Read the model definition and answer for the solid it produces. Units are mm, in the model's axes. A direction names the side the tool comes from. Give positions to 0.01 mm unless a question says otherwise; leave off trailing zeros. Write each loop counter-clockwise with the first axis right and the second up, starting at its lowest first coordinate (ties: lowest second). Pieces come first, ordered by that corner, then holes. Notation, with made-up numbers: (79.5, -9.75) - (136.5, -9.75) arc R33 cw to (136.5, 27.25) - close; hole circle Ø3 at (-18, 61.5). An arc over 180 degrees is marked (long way). Answer as a JSON object with one key per item and string values. Group by question number.
```python
from build123d import *

# Parameters (mm, degrees)
BOSS_EXTRUDE1_DEPTH     = 2
CUT_EXTRUDE1_DEPTH      = 6.766281297
CUT_EXTRUDE1_DEPTH_BACK = 6.766281297
SKETCH2_R               = 1.55
BOSS_EXTRUDE2_START     = 4.6
BOSS_EXTRUDE2_DEPTH     = 4.6
BOSS_EXTRUDE3_DEPTH     = 2
FILLET1_R               = 0.5


with BuildPart() as part:
    # Sketch1 → Boss-Extrude1 (new body)
    with BuildSketch(Plane(origin=(0, 0, 0), x_dir=(1, 0, 0), z_dir=(0, 1, 0))):
        with BuildLine():
            Line((2.5, 3), (-2.5, 3))
            ThreePointArc((-2.5, 3), (-3.914213562, 2.414213562), (-4.5, 1))
            Line((-4.5, 1), (-4.5, -1))
            ThreePointArc((-4.5, -1), (-3.914213562, -2.414213562), (-2.5, -3))
            Line((-2.5, -3), (2.5, -3))
            ThreePointArc((2.5, -3), (3.914213562, -2.414213562), (4.5, -1))
            Line((4.5, -1), (4.5, 1))
            ThreePointArc((4.5, 1), (3.914213562, 2.414213562), (2.5, 3))
        make_face()
    extrude(amount=BOSS_EXTRUDE1_DEPTH)

    # Sketch2 → Cut-Extrude1 (cut, two sides: drawn at the far end of the back side and taken through both)
    with BuildSketch(Plane(origin=(0, 2, 0), x_dir=(1, 0, 0), z_dir=(0, 1, 0)).offset(-CUT_EXTRUDE1_DEPTH_BACK)):
        with Locations(Location((-1.6, 0, 0), (0, 0, 270))):
            Circle(SKETCH2_R)
    extrude(amount=CUT_EXTRUDE1_DEPTH + CUT_EXTRUDE1_DEPTH_BACK, mode=Mode.SUBTRACT)

    # Sketch3 → Boss-Extrude2 (add)
    with BuildSketch(Plane.XZ.offset(BOSS_EXTRUDE2_START)):
        with BuildLine():
            Line((4.5, 1), (4.5, -1))
            ThreePointArc((4.5, -1), (3.914213562, -2.414213562), (2.5, -3))
            Line((2.5, -3), (2.5, 3))
            ThreePointArc((2.5, 3), (3.914213562, 2.414213562), (4.5, 1))
        make_face()
    extrude(amount=-BOSS_EXTRUDE2_DEPTH)

    # Sketch4 → Boss-Extrude3 (add)
    with BuildSketch(Plane.XZ.offset(4.6)):
        with BuildLine():
            Line((4.5, 1), (4.5, -1))
            ThreePointArc((4.5, -1), (3.914213562, -2.414213562), (2.5, -3))
            Line((2.5, -3), (5.5, -3))
            ThreePointArc((5.5, -3), (6.560660172, -2.560660172), (7, -1.5))
            Line((7, -1.5), (7, 1.5))
            ThreePointArc((7, 1.5), (6.560660172, 2.560660172), (5.5, 3))
            Line((5.5, 3), (2.5, 3))
            ThreePointArc((2.5, 3), (3.914213562, 2.414213562), (4.5, 1))
        make_face()
    extrude(amount=-BOSS_EXTRUDE3_DEPTH)

    # Fillet1
    # the kernel refuses this fillet: 0.5 mm, written as the material it takes off along each edge
    with BuildSketch(Plane(origin=(-2.5, 2, 1), x_dir=(-1, 0, 0), z_dir=(0, 0, -1))) as fillet1_piece_1:
        with BuildLine():
            CenterArc((2 - FILLET1_R, -FILLET1_R), FILLET1_R, 0, 90)
            Line((2, -FILLET1_R), (2, 0))
            Line((2, 0), (2 - FILLET1_R, 0))
        make_face()
    revolve(axis=Axis((-2.5, 2, 1), (0, 1, 0)), revolution_arc=90, mode=Mode.SUBTRACT)
    with BuildSketch(Plane(origin=(-2.5, 2, 3), x_dir=(0, 0, -1), z_dir=(1, 0, 0)), Plane(origin=(2.5, 2, -3), x_dir=(0, 0, 1), z_dir=(-1, 0, 0))) as fillet1_piece_2:
        with BuildLine():
            CenterArc((FILLET1_R, -FILLET1_R), FILLET1_R, 90, 90)
            Line((0, -FILLET1_R), (0, 0))
            Line((0, 0), (FILLET1_R, 0))
        make_face()
    extrude(amount=5, mode=Mode.SUBTRACT)
    with BuildSketch(Plane(origin=(2.5, 2, 1), x_dir=(0, 0, 1), z_dir=(-1, 0, 0))) as fillet1_piece_3:
        with BuildLine():
            CenterArc((2 - FILLET1_R, -FILLET1_R), FILLET1_R, 0, 90)
            Line((2 - FILLET1_R, 0), (2, 0))
            Line((2, 0), (2, -FILLET1_R))
        make_face()
    revolve(axis=Axis((2.5, 2, 1), (0, 1, 0)), revolution_arc=90, mode=Mode.SUBTRACT)
    with BuildSketch(Plane(origin=(4.5, 2, 1), x_dir=(0, -1, 0), z_dir=(0, 0, -1))) as fillet1_piece_4:
        with BuildLine():
            CenterArc((FILLET1_R, FILLET1_R), FILLET1_R, 180, 90)
            Line((0, FILLET1_R), (0, 0))
            Line((0, 0), (FILLET1_R, 0))
        make_face()
    extrude(amount=2, mode=Mode.SUBTRACT)
    with BuildSketch(Plane(origin=(-1.6, 0, 0), x_dir=(0, 0, 1), z_dir=(-1, 0, 0))) as fillet1_piece_5:
        with BuildLine():
            CenterArc((1.55 + FILLET1_R, FILLET1_R), FILLET1_R, 180, 90)
            Line((1.55 + FILLET1_R, 0), (1.55, 0))
            Line((1.55, 0), (1.55, FILLET1_R))
        make_face()
    revolve(axis=Axis((-1.6, 0, 0), (0, 1, 0)), mode=Mode.SUBTRACT)
    with BuildSketch(Plane(origin=(2.5, 2, -1), x_dir=(1, 0, 0), z_dir=(0, 0, 1))) as fillet1_piece_6:
        with BuildLine():
            CenterArc((2 - FILLET1_R, -FILLET1_R), FILLET1_R, 0, 90)
            Line((2 - FILLET1_R, 0), (2, 0))
            Line((2, 0), (2, -FILLET1_R))
        make_face()
    revolve(axis=Axis((2.5, 2, -1), (0, 1, 0)), revolution_arc=90, mode=Mode.SUBTRACT)
    with BuildSketch(Plane(origin=(5.5, -2.6, 3), x_dir=(0, 0, -1), z_dir=(-1, 0, 0))) as fillet1_piece_7_section:
        with BuildLine():
            CenterArc((FILLET1_R, FILLET1_R), FILLET1_R, 180, 90)
            Line((0, FILLET1_R), (0, 0))
            Line((0, 0), (FILLET1_R, 0))
        make_face()
    fillet1_piece_7 = extrude(amount=4.25, mode=Mode.PRIVATE)
    fillet1_piece_7 = fillet1_piece_7 - Plane(origin=(2.5, -2.684531393, 1), x_dir=(0, 0, 1), z_dir=(0, -1, 0)) * Cylinder(2, 11, mode=Mode.PRIVATE)
    add(fillet1_piece_7, mode=Mode.SUBTRACT)
    with BuildSketch(Plane(origin=(5.5, -2.6, 1.5), x_dir=(1, 0, 0), z_dir=(0, 0, -1))) as fillet1_piece_8:
        with BuildLine():
            CenterArc((1.5 - FILLET1_R, FILLET1_R), FILLET1_R, 270, 90)
            Line((1.5, FILLET1_R), (1.5, 0))
            Line((1.5, 0), (1.5 - FILLET1_R, 0))
        make_face()
    revolve(axis=Axis((5.5, -2.6, 1.5), (0, -1, 0)), revolution_arc=90, mode=Mode.SUBTRACT)
    with BuildSketch(Plane(origin=(7, -2.6, -1.5), x_dir=(-1, 0, 0), z_dir=(0, 0, 1))) as fillet1_piece_9:
        with BuildLine():
            CenterArc((FILLET1_R, FILLET1_R), FILLET1_R, 180, 90)
            Line((0, FILLET1_R), (0, 0))
            Line((0, 0), (FILLET1_R, 0))
        make_face()
    extrude(amount=3, mode=Mode.SUBTRACT)
    with BuildSketch(Plane(origin=(5.5, -2.6, -1.5), x_dir=(0, 0, -1), z_dir=(-1, 0, 0))) as fillet1_piece_10:
        with BuildLine():
            CenterArc((1.5 - FILLET1_R, FILLET1_R), FILLET1_R, 270, 90)
            Line((1.5, FILLET1_R), (1.5, 0))
            Line((1.5, 0), (1.5 - FILLET1_R, 0))
        make_face()
    revolve(axis=Axis((5.5, -2.6, -1.5), (0, -1, 0)), revolution_arc=90, mode=Mode.SUBTRACT)
    with BuildSketch(Plane(origin=(1.25, -2.6, -3), x_dir=(0, 0, 1), z_dir=(1, 0, 0))) as fillet1_piece_11_section:
        with BuildLine():
            CenterArc((FILLET1_R, FILLET1_R), FILLET1_R, 180, 90)
            Line((0, FILLET1_R), (0, 0))
            Line((0, 0), (FILLET1_R, 0))
        make_face()
    fillet1_piece_11 = extrude(amount=4.25, mode=Mode.PRIVATE)
    fillet1_piece_11 = fillet1_piece_11 - Plane(origin=(2.5, -2.72746411, -1), x_dir=(1, 0, 0), z_dir=(0, -1, 0)) * Cylinder(2, 11, mode=Mode.PRIVATE)
    add(fillet1_piece_11, mode=Mode.SUBTRACT)
    with BuildSketch(Plane(origin=(-2.5, 2, -1), x_dir=(0, 0, -1), z_dir=(1, 0, 0))) as fillet1_piece_12:
        with BuildLine():
            CenterArc((2 - FILLET1_R, -FILLET1_R), FILLET1_R, 0, 90)
            Line((2, -FILLET1_R), (2, 0))
            Line((2, 0), (2 - FILLET1_R, 0))
        make_face()
    revolve(axis=Axis((-2.5, 2, -1), (0, 1, 0)), revolution_arc=90, mode=Mode.SUBTRACT)
    with BuildSketch(Plane(origin=(-4.5, 2, -1), x_dir=(1, 0, 0), z_dir=(0, 0, 1))) as fillet1_piece_13:
        with BuildLine():
            CenterArc((FILLET1_R, -FILLET1_R), FILLET1_R, 90, 90)
            Line((0, -FILLET1_R), (0, 0))
            Line((0, 0), (FILLET1_R, 0))
        make_face()
    extrude(amount=2, mode=Mode.SUBTRACT)


solid = part.part
```
1) Flat-ended cylindrical pins translate along their axes: pin 1 Ø3 at (x, z) = (-1, -0.5) entering from -Y; pin 2 Ø2 at (y, z) = (-0.5, 0.5) entering from +X; pin 3 Ø3.5 at (y, z) = (-2.5, -1.5) entering from -X. Find the tip coordinate at first contact, or state that the pin passes through.
2) Find section C-C, the plane x = 1. Write down the section's boundary in (y, z), and give its area (3 significant figures).
3) Find section B-B, the plane z = 0. Write down the section's boundary in (x, y), and give its area (3 significant figures).
4) Which of the six approach directions +Z, -Z, +X, -X, +Y, -Y give full straight-line access (tool end or side, diameter ignored) to faces 1 (the flat face through (4.5, -1, 0)), 2 (the flat face through (2.5, -2, 0)), 3 (the cylindrical face through (-3.93, 0.74, 2.4))?
5) Find section A-A, the plane x = -1.6. Write down the section's boundary in (y, z).
6) Find the intervals of material crossed by line 1 (X direction, y = 0.9, z = 0); line 2 (Z direction, x = -1.6, y = 1.5); line 3 (Y direction, x = -2.75, z = -1.75), in increasing order. Write a range as [from, to].
7) For a pull along Z with two mould halves and no side action, classify faces 4 (the cylindrical face through (-3.9, 0.74, -2.43)), 5 (the cylindrical face through (-1.134, 1.24, 1.478)), 6 (the cylindrical face through (6.57, -3.86, 2.55)), 7 (the flat face through (-4.5, 1, 0)) as released by +Z, released by -Z, zero draft, split by the parting line, or undercut.
8) Find section D-D, the plane y = -0.5. Write down the section's boundary in (x, z).
Values follow:
{
 "1": {"pin 1": "stops at y = 0", "pin 2": "stops at x = 4.5", "pin 3": "stops at x = 2.5"},
 "2": {"outline": "(0, -3) - (1.5, -3) arc R0.5 ccw to (2, -2.5) - (2, 2.5) arc R0.5 ccw to (1.5, 3) - (0, 3) - close", "area": "11.9 mm2"},
 "3": {"outline": "(-4.5, 0) - (-3.65, 0) arc R0.5 ccw to (-3.15, 0.5) - (-3.15, 2) - (-4, 2) arc R0.5 ccw to (-4.5, 1.5) - close; (-0.05, 0.5) arc R0.5 ccw to (0.45, 0) - (2.5, 0) - (2.5, -4.6) - (7, -4.6) - (7, -3.1) arc R0.5 ccw to (6.5, -2.6) - (4.5, -2.6) - (4.5, 1.5) arc R0.5 ccw to (4, 2) - (-0.05, 2) - close", "area": "25.7 mm2"},
 "4": {"face 1": "+Z, -Z, +X, +Y", "face 2": "+Z, -Z, -X, -Y", "face 3": "+Z, -X, +Y, -Y"},
 "5": {"outline": "(0, -3) - (1.5, -3) arc R0.5 ccw to (2, -2.5) - (2, -1.55) - (0.5, -1.55) arc R0.5 ccw to (0, -2.05) - close; (0, 2.05) arc R0.5 ccw to (0.5, 1.55) - (2, 1.55) - (2, 2.5) arc R0.5 ccw to (1.5, 3) - (0, 3) - close"},
 "6": {"line 1": "x = [-4.5, -3.15], [-0.05, 4.5]", "line 2": "z = [-3, -1.55], [1.55, 3]", "line 3": "y = [0, 2]"},
 "7": {"face 4": "released by -Z", "face 5": "undercut", "face 6": "released by +Z", "face 7": "zero draft"},
 "8": {"outline": "(2.5, -3) arc R2 ccw to (4.5, -1) - (4.5, 1) arc R2 ccw to (2.5, 3) - close"}
}
